```python
from build123d import *

# Parameters (mm, degrees)
BOSS_EXTRUDE1_DEPTH          = 19.05
SKETCH1_3_R                  = 9.525
BOSS_EXTRUDE2_DEPTH          = 20.828
CHAMFER1_SIZE                = 1.524
BOSS_EXTRUDE3_START          = -19.05
SKETCH1_4_R                  = 19.05
BOSS_EXTRUDE3_DEPTH          = 44.45
BOSS_EXTRUDE4_START          = -19.05
SKETCH1_6_R                  = 25.4
SKETCH1_6_R_2                = 19.05
BOSS_EXTRUDE4_DEPTH          = 19.05
BOSS_EXTRUDE5_START          = 76.2
SKETCH1_7_R                  = 19.05
BOSS_EXTRUDE5_DEPTH          = 76.2
BOSS_EXTRUDE6_START          = 107.95
SKETCH1_8_R                  = 50.8
SKETCH1_8_R_2                = 25.4
SKETCH1_8_R_3                = 19.05
BOSS_EXTRUDE6_DEPTH          = 31.75
CIRPATTERN2_COUNT            = 2
CHAMFER1_OF_CIRPATTERN2_SIZE = 1.524
FILLET1_R                    = 12.7
CUT_REVOLVE1_START           = 34.798
CUT_REVOLVE1_OUTLINE_R       = 6.35
CUT_REVOLVE1_DEPTH           = 16.0020001
CIRPATTERN3_COUNT            = 4


# Read off the part's stored shape, not the designer's step: Cut-Revolve1
with BuildPart() as part:
    # Sketch1 → Boss-Extrude1 (new body)
    with BuildSketch(Plane.YZ):
        with BuildLine():
            ThreePointArc((-101.152530245, -9.525), (0, -101.6), (101.152530245, -9.525))
            Line((101.152530245, -9.525), (82.55, -9.525))
            Line((82.55, -9.525), (82.55, 9.525))
            Line((82.55, 9.525), (101.152530245, 9.525))
            ThreePointArc((101.152530245, 9.525), (0, 101.6), (-101.152530245, 9.525))
            Line((-101.152530245, 9.525), (-82.55, 9.525))
            Line((-82.55, 9.525), (-82.55, -9.525))
            Line((-82.55, -9.525), (-101.152530245, -9.525))
        make_face()
    extrude(amount=-BOSS_EXTRUDE1_DEPTH)

    # Sketch1<3> → Boss-Extrude2 (add)
    with BuildSketch(Plane.YZ):
        with Locations(Location((0, 76.2, 0), (0, 0, 270))):
            Circle(SKETCH1_3_R)
    boss_extrude2 = extrude(amount=BOSS_EXTRUDE2_DEPTH)

    # Chamfer1
    chamfer1_edges = [part.edges().sort_by_distance(p)[0] for p in [
        (20.828, 0, 85.725),
    ]]
    chamfer(chamfer1_edges, length=CHAMFER1_SIZE)

    # Sketch1<4> → Boss-Extrude3 (add)
    with BuildSketch(Plane.YZ.offset(BOSS_EXTRUDE3_START)):
        with Locations(Location((0, 0, 0), (0, 0, 270))):
            Circle(SKETCH1_4_R)
    extrude(amount=-BOSS_EXTRUDE3_DEPTH)

    # Sketch1<6> → Boss-Extrude4 (add)
    with BuildSketch(Plane.YZ.offset(BOSS_EXTRUDE4_START)):
        with Locations(Location((0, 0, 0), (0, 0, 90))):
            Circle(SKETCH1_6_R)
        with Locations(Location((0, 0, 0), (0, 0, 270))):
            Circle(SKETCH1_6_R_2, mode=Mode.SUBTRACT)
    extrude(amount=-BOSS_EXTRUDE4_DEPTH)

    # Sketch1<7> → Boss-Extrude5 (add)
    with BuildSketch(Plane.YZ.offset(BOSS_EXTRUDE5_START)):
        with Locations(Location((0, 0, 0), (0, 0, 270))):
            Circle(SKETCH1_7_R)
    extrude(amount=-BOSS_EXTRUDE5_DEPTH)

    # Sketch1<8> → Boss-Extrude6 (add)
    # profile 1 of 3: a face of its own
    with BuildSketch(Plane.YZ.offset(BOSS_EXTRUDE6_START)):
        with Locations(Location((0, 0, 0), (0, 0, 270))):
            Circle(SKETCH1_8_R)
        with Locations(Location((0, 0, 0), (0, 0, 90))):
            Circle(SKETCH1_8_R_2, mode=Mode.SUBTRACT)
    # profile 2 of 3: a face of its own
    with BuildSketch(Plane.YZ.offset(BOSS_EXTRUDE6_START)):
        with Locations(Location((0, 0, 0), (0, 0, 90))):
            Circle(SKETCH1_8_R_2)
        with Locations(Location((0, 0, 0), (0, 0, 270))):
            Circle(SKETCH1_8_R_3, mode=Mode.SUBTRACT)
    # profile 3 of 3: a face of its own
    with BuildSketch(Plane.YZ.offset(BOSS_EXTRUDE6_START)):
        with Locations(Location((0, 0, 0), (0, 0, 270))):
            Circle(SKETCH1_8_R_3)
    extrude(amount=-BOSS_EXTRUDE6_DEPTH)

    # CirPattern2: Boss-Extrude2 ×2 about axis
    cirpattern2_axis = Axis((0, 0, 0), (1, 0, 0))
    for i in range(1, CIRPATTERN2_COUNT):
        add(boss_extrude2.rotate(cirpattern2_axis, i * 360 / CIRPATTERN2_COUNT))

    # Chamfer1 of CirPattern2
    chamfer1_of_cirpattern2_edges = [part.edges().sort_by_distance(p)[0] for p in [
        (20.828, 0, -85.725),
    ]]
    chamfer(chamfer1_of_cirpattern2_edges, length=CHAMFER1_OF_CIRPATTERN2_SIZE)

    # Fillet1
    fillet1_edges = [part.edges().sort_by_distance(p)[0] for p in [
        (107.95, 0, 50.8),
    ]]
    fillet(fillet1_edges, radius=FILLET1_R)

    # Cut-Revolve1 outline → Cut-Revolve1 (cut)
    with BuildSketch(Plane(origin=(0, 0, 0), x_dir=(1, 0, 0), z_dir=(0, 0.707106781186549, -0.707106781186546)).offset(CUT_REVOLVE1_START)):
        with Locations((88.9, 0)):
            Circle(CUT_REVOLVE1_OUTLINE_R)
    cut_revolve1 = extrude(amount=CUT_REVOLVE1_DEPTH, mode=Mode.SUBTRACT)

    # CirPattern3: Cut-Revolve1 ×4 about axis
    cirpattern3_axis = Axis((0, 0, 0), (1, 0, 0))
    for i in range(1, CIRPATTERN3_COUNT):
        add(cut_revolve1.rotate(cirpattern3_axis, i * 360 / CIRPATTERN3_COUNT), mode=Mode.SUBTRACT)


solid = part.part
```
The listing builds one solid part. Answer for the finished solid, in the listing's coordinates (mm). A direction names the side the tool comes from. Round coordinates to 2 decimals unless told otherwise and drop trailing zeros. Loops run counter-clockwise (first coordinate to the right, second up) from the corner with the lowest first, then second, coordinate; pieces in that order, holes last.
Q1. Section A-A, the plane z = 0 is taken. Determine the outline of the cut face in (x, y), then the cut area to 3 significant figures.
Q2. Find the intervals of material crossed by line 1 (X direction, y = 21.5, z = 88.5); line 2 (Y direction, x = 50.5, z = 17); line 3 (Z direction, x = -29, y = 8), in increasing order.
Q3. Section C-C, the plane x = 90 is taken. Determine the outline of the cut face in (y, z).
Q4. Which of the six approach directions +Z, -Z, +X, -X, +Y, -Y give full straight-line access (tool end or side, diameter ignored) to faces 4 (the face through (-9, 92, -9.525)), 5 (the face through (76.2, 1, -22)), 6 (the face through (9.517, -0.419, -85.716))?
Q5. Section D-D, the plane z = 76.2 is taken. Determine the outline of the cut face in (x, y) (3 decimals), then the cut area to 3 significant figures.
Q6. For a pull along X with two mould halves and no side action, classify faces 1 (the face through (-63.5, 0, 0)), 2 (the face through (88.81, 24.54, -24.67)), 3 (the face through (-50.62, -11.59, 15.12)) as released by +X, released by -X, zero draft, split by the parting line, or undercut.
Q7. Given pin 1 Ø20.5 at (x, y) = (-13, 96) entering from -Z; pin 2 Ø8 at (y, z) = (0, 78.5) entering from +X; pin 3 Ø10 at (x, y) = (38, 9) entering from -Z; pin 4 Ø12 at (x, y) = (22.5, 31) entering from -Z, each flat-ended and moving along its own axis, determine where each tip first touches the part or whether it passes through.
Completed:
1. outline: (-63.5, -19.05) - (-38.1, -19.05) - (-38.1, -25.4) - (-19.05, -25.4) - (-19.05, -82.55) - (0, -82.55) - (0, -19.05) - (76.2, -19.05) - (76.2, -50.8) - (95.25, -50.8) arc R12.7 ccw to (107.95, -38.1) - (107.95, 38.1) arc R12.7 ccw to (95.25, 50.8) - (76.2, 50.8) - (76.2, 19.05) - (0, 19.05) - (0, 82.55) - (-19.05, 82.55) - (-19.05, 25.4) - (-38.1, 25.4) - (-38.1, 19.05) - (-63.5, 19.05) - close
1. area: 11,100 mm2
2. line 1: x = -19.05 to 0
2. line 2: y = -8.6 to 8.6
2. line 3: z = -24.11 to 24.11
3. outline: (-40.07, -31.23) - (-29.03, -20.18) - (-20.18, -29.03) - (-31.23, -40.07) arc R50.8 ccw to (31.23, -40.07) - (20.18, -29.03) - (29.03, -20.18) - (40.07, -31.23) arc R50.8 ccw to (40.07, 31.23) - (29.03, 20.18) - (20.18, 29.03) - (31.23, 40.07) arc R50.8 ccw to (-31.23, 40.07) - (-20.18, 29.03) - (-29.03, 20.18) - (-40.07, 31.23) arc R50.8 ccw to start
4. face 4: +X, -X, +Y
4. face 5: none
4. face 6: +X
5. outline: (-19.05, -67.202) - (0, -67.202) - (0, -9.525) - (19.304, -9.525) - (20.828, -8.001) - (20.828, 8.001) - (19.304, 9.525) - (0, 9.525) - (0, 67.202) - (-19.05, 67.202) - close
5. area: 2,950 mm2
6. face 1: released by -X
6. face 2: undercut
6. face 3: zero draft
7. pin 1: stops at z = -54.49
7. pin 2: stops at x = 20.83
7. pin 3: stops at z = -18.63
7. pin 4: passes through
